Work out the finished part from the listing and answer in its coordinate system (mm). A direction names the side the tool comes from. Give positions to 0.01 mm unless a question says otherwise; leave off trailing zeros. Order: outer loops, then holes, each group sorted by start corner. A loop starts at its lowest first (then second) coordinate and runs counter-clockwise, first axis right, second up. Notation, with made-up numbers: (-16, 41) - (26, 41) arc R22 ccw to (26, 52) - close; hole circle Ø8 at (-10.5, -18). An arc over 180 degrees is marked (long way). Put each result on its own line as item: value.
```python
from build123d import *

# Parameters (mm, degrees)
SKETCH1_R           = 3.25
SKETCH1_R_2         = 4.25
SKETCH1_R_3         = 7
BOSS_EXTRUDE1_DEPTH = 10
SKETCH2_R           = 1.5
CUT_EXTRUDE1_DEPTH  = 10
FILLET1_R           = 10


with BuildPart() as part:
    # Sketch1 → Boss-Extrude1 (new body)
    with BuildSketch(Plane.XY):
        with BuildLine():
            Line((5.110545705, -6.47648227), (45, 25))
            Line((45, 25), (45, 47))
            Line((45, 47), (27, 47))
            Line((27, 47), (-6.444784556, 5.150461341))
            ThreePointArc((-6.444784556, 5.150461341), (-5.851623942, -5.815582279), (5.110545705, -6.47648227))
        make_face()
        Circle(SKETCH1_R, mode=Mode.SUBTRACT)
        with Locations((30, 30)):
            Circle(SKETCH1_R_2, mode=Mode.SUBTRACT)
        with Locations((15, 15)):
            Circle(SKETCH1_R_3, mode=Mode.SUBTRACT)
    extrude(amount=BOSS_EXTRUDE1_DEPTH)

    # Sketch2 → Cut-Extrude1 (cut)
    with BuildSketch(Plane(origin=(45, 0, 0), x_dir=(0, 0, -1), z_dir=(1, 0, 0))):
        with Locations((-5, 43)):
            Circle(SKETCH2_R)
        with Locations((-5, 35)):
            Circle(SKETCH2_R)
    extrude(amount=-CUT_EXTRUDE1_DEPTH, mode=Mode.SUBTRACT)

    # Fillet1
    fillet1_edges = [part.edges().sort_by_distance(p)[0] for p in [
        (27, 47, 5),
    ]]
    fillet(fillet1_edges, radius=FILLET1_R)


solid = part.part
```
(1) Given pin 1 (2 mm diameter, centred on y = 21.5, z = 9, fed in from +X); pin 2 (1 mm diameter, centred on y = 34.5, z = 4.5, fed in from +X); pin 3 (3 mm diameter, centred on y = 8, z = 6, fed in from -X), each flat-ended and moving along its own axis, determine where each tip first touches the part or whether it passes through.
Geometry check:
pin 1: stops at x = 41.83
pin 2: stops at x = 35
pin 3: stops at x = -5.37
(2) A tool of negligible diameter and unlimited length cuts with its end or side. For faces 5 (the face through (24, 20, 10)), 6 (the face through (35, 43, 5)), from which of +Z, -Z, +X, -X, +Y, -Y can it reach the whole face along a straight path? Write none if from no direction.
Geometry check:
face 5: +Z, +X, -X, +Y, -Y
face 6: +X
(3) Section B-B, the plane y = 13.5 is taken. Write down the section's boundary in (x, z), then the cut area to 3 significant figures.
Geometry check:
outline: (0.23, 0) - (8.16, 0) - (8.16, 10) - (0.23, 10) - close; (21.84, 0) - (30.43, 0) - (30.43, 10) - (21.84, 10) - close
area: 165 mm²
(4) Section D-D, the plane z = 1.5 is taken. Write down the section's boundary in (x, y).
Geometry check:
outline: (-6.44, 5.15) arc R8.25 ccw to (5.11, -6.48) - (45, 25) - (45, 47) - (31.81, 47) arc R10 ccw to (24, 43.24) - close; hole circle Ø6.5 at (0, 0); hole circle Ø14 at (15, 15); hole circle Ø8.5 at (30, 30)
(5) Section A-A, the plane z = 5 is taken. Write down the section's boundary in (x, y).
Geometry check:
outline: (-6.44, 5.15) arc R8.25 ccw to (5.11, -6.48) - (45, 25) - (45, 33.5) - (35, 33.5) - (35, 36.5) - (45, 36.5) - (45, 41.5) - (35, 41.5) - (35, 44.5) - (45, 44.5) - (45, 47) - (31.81, 47) arc R10 ccw to (24, 43.24) - close; hole circle Ø6.5 at (0, 0); hole circle Ø14 at (15, 15); hole circle Ø8.5 at (30, 30)
(6) Straight lines are drawn through the part: line 1 (Y direction, x = 42.5, z = 5); line 2 (X direction, y = 9, z = 9.5); line 3 (Y direction, x = 37.5, z = 5). For each, find the intervals that lie inside material, in ascending order.
Geometry check:
line 1: y = 23.03 to 33.5, 36.5 to 41.5, 44.5 to 47
line 2: x = -3.37 to 11.39, 18.61 to 24.72
line 3: y = 19.08 to 33.5, 36.5 to 41.5, 44.5 to 47
(7) Determine the mould class of faces 1 (the face through (40.07, 41.536, 5.325)), 2 (the face through (24, 20, 0)), 3 (the face through (35, 35, 5)), 4 (the face through (38, 47, 5)) for opening direction Z: pulls with the +Z half, pulls with the -Z half, needs draft (parallel to the pull), parting line crosses it, or undercut.
Geometry check:
face 1: undercut
face 2: pulls with the -Z half
face 3: undercut
face 4: needs draft
(8) Section C-C, the plane x = 12.5 is taken. Write down the section's boundary in (y, z).
Geometry check:
outline: (-0.65, 0) - (8.46, 0) - (8.46, 10) - (-0.65, 10) - close; (21.54, 0) - (28.86, 0) - (28.86, 10) - (21.54, 10) - close
